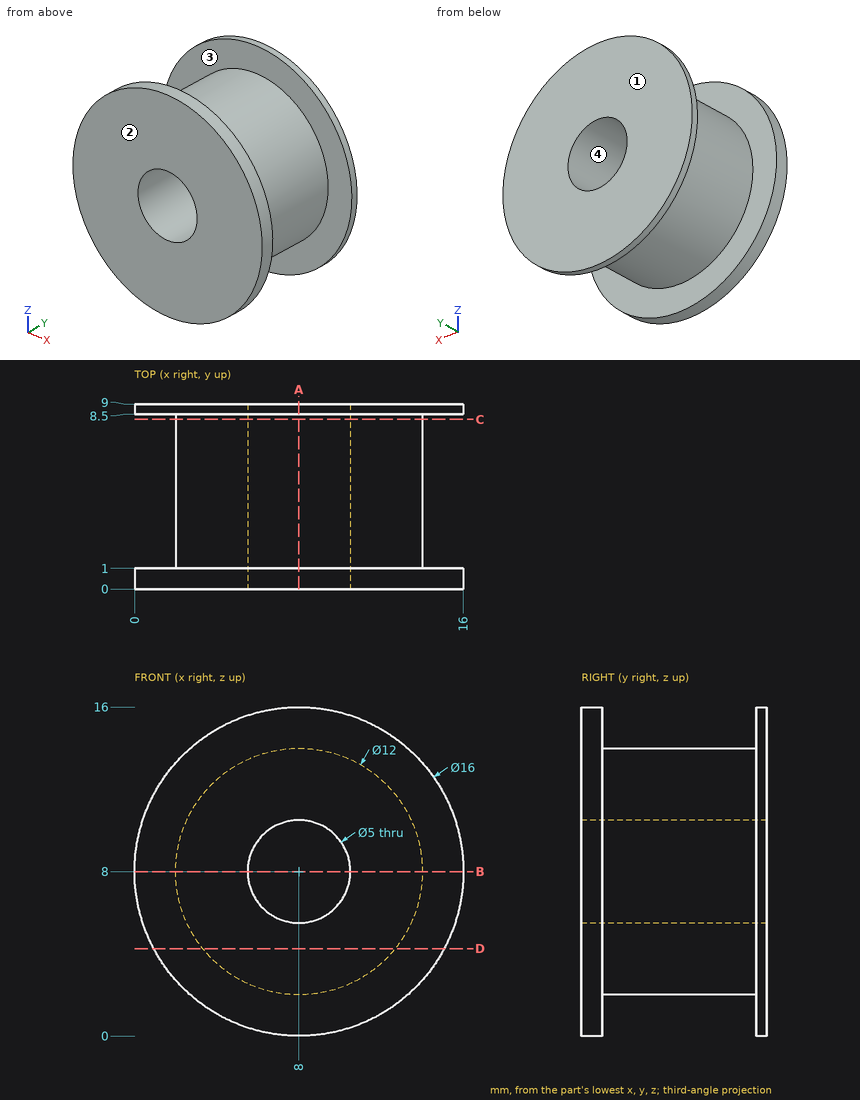
Drawing for the job (mm, zero at the part's lowest x, y, z). Give positions to 0.01 mm unless a question says otherwise; leave off trailing zeros. Order: outer loops, then holes, each group sorted by start corner. A loop starts at its lowest first (then second) coordinate and runs counter-clockwise, first axis right, second up. Notation, with made-up numbers: M -11.5,47.25 L 12.5,47.25 A22 ccw 12.5,54.25 Z; hole C 78,40.5 d10. An arc over 180 degrees is marked long. Put each result on its own line as item: value.
Item 1: Slice it at A-A, the plane x = 8. Write the cut outline in (y, z), plus the area to 3 significant figures.
From the geometry:
outline: M 0,0 L 1,0 L 1,2 L 8.5,2 L 8.5,0 L 9,0 L 9,5.5 L 0,5.5 Z; M 0,10.5 L 9,10.5 L 9,16 L 8.5,16 L 8.5,14 L 1,14 L 1,16 L 0,16 Z
area: 69.0 mm2
Item 2: Slice it at B-B, the plane z = 8. Write the cut outline in (x, y).
From the geometry:
outline: M 0,0 L 5.5,0 L 5.5,9 L 0,9 L 0,8.5 L 2,8.5 L 2,1 L 0,1 Z; M 10.5,0 L 16,0 L 16,1 L 14,1 L 14,8.5 L 16,8.5 L 16,9 L 10.5,9 Z
Item 3: Slice it at C-C, the plane y = 8.25. Write the cut outline in (x, z), plus the area to 3 significant figures.
From the geometry:
outline: C 8,8 d12; hole C 8,8 d5
area: 93.5 mm2
Item 4: Slice it at D-D, the plane z = 4.25. Write the cut outline in (x, y).
From the geometry:
outline: M 0.93,0 L 15.07,0 L 15.07,1 L 12.68,1 L 12.68,8.5 L 15.07,8.5 L 15.07,9 L 0.93,9 L 0.93,8.5 L 3.32,8.5 L 3.32,1 L 0.93,1 Z
Item 5: Two-plate mould, pull along Y, no slides. Class the marked faces 1, 2, 3 and 4: +Y half, -Y half, draft (parallel to the pull), parting line (faces both ways), or undercut.
From the geometry:
face 1: +Y half
face 2: -Y half
face 3: undercut
face 4: draft
Item 6: Probe line 1 (Y direction, x = 3.5, z = 3.5); line 2 (X direction, y = 2, z = 8); line 3 (Z direction, x = 8.75, y = 5.75). List the from-to ranges inside material, lowest first. Write a range as [from, to].
From the geometry:
line 1: y = [0, 1], [8.5, 9]
line 2: x = [2, 5.5], [10.5, 14]
line 3: z = [2.05, 5.62], [10.38, 13.95]
Item 7: Flat gauge pins, fed straight in: pin 1 Ø3 at (y, z) = (3.5, 9.5) entering from +X; pin 2 Ø1.5 at (x, y) = (7.5, 2) entering from -Z; pin 3 Ø3 at (x, y) = (12, 3.5) entering from +Z. Where does each tip first touch, or does it go through?
From the geometry:
pin 1: stops at x = 14
pin 2: stops at z = 2
pin 3: stops at z = 13.45
